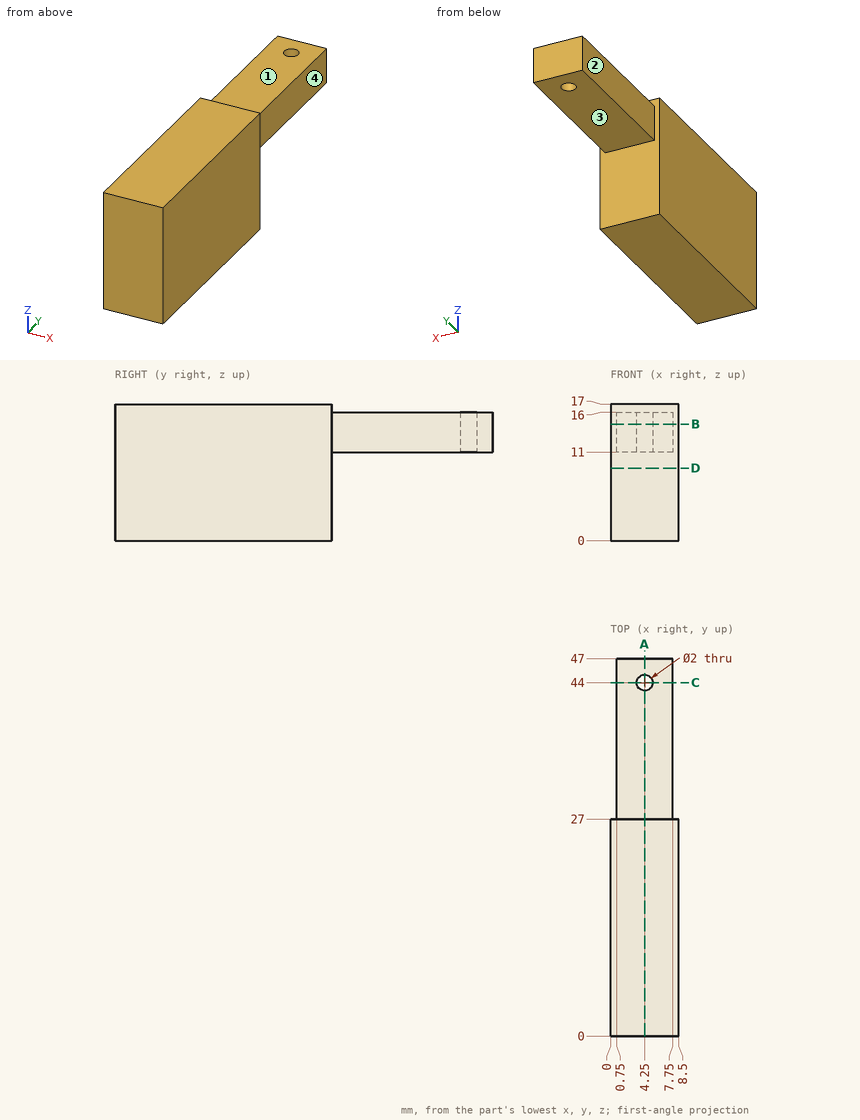
Answer from the drawing. Dimensions are ordinates in mm from the lowest x, y and z of the part. A direction names the side the tool comes from. Give positions to 0.01 mm unless a question says otherwise; leave off trailing zeros. Write each loop counter-clockwise with the first axis right and the second up, starting at its lowest first coordinate (ties: lowest second). Pieces come first, ordered by that corner, then holes. Notation, with made-up numbers: (75, -39.75) - (117, -39.75) arc R36 ccw to (117, -5.75) - close; hole circle Ø3 at (38, -23). An arc over 180 degrees is marked (long way). One line per item, written item: value. Start each with the question number.
1. Find section A-A (x = 4.25). Write down the section's boundary in (y, z), then the cut area to 3 significant figures.
2. Find section C-C (y = 44). Write down the section's boundary in (x, z), then the cut area to 3 significant figures.
3. Find section B-B (z = 14.5). Write down the section's boundary in (x, y).
4. Find section D-D (z = 9). Write down the section's boundary in (x, y).
5. Consider probe 1 along Y at (x, z) = (4.25, 13.3); probe 2 along Z at (x, y) = (7.25, 38.5); probe 3 along Y at (x, z) = (4.25, 1.5). Determine where each line is inside the solid, lowest interval first.
6. For the marked faces 1, 2, 3 and 4, determine the directions among +Z, -Z, +X, -X, +Y, -Y from which every point of the face is accessible in a straight line to the end or side of a thin tool.
7. Given pin 1 (1 mm diameter, centred on x = 5.5, y = 5, fed in from -Z); pin 2 (4 mm diameter, centred on x = 3.5, z = 8.5, fed in from +Y); pin 3 (4 mm diameter, centred on x = 4, y = 30, fed in from +Z); pin 4 (1.5 mm diameter, centred on y = 37.5, z = 13, fed in from -X), each flat-ended and moving along its own axis, determine where each tip first touches the part or whether it passes through.
Geometry results:
1. outline: (0, 0) - (27, 0) - (27, 11) - (43, 11) - (43, 16) - (27, 16) - (27, 17) - (0, 17) - close; (45, 11) - (47, 11) - (47, 16) - (45, 16) - close
1. area: 549 mm2
2. outline: (0.75, 11) - (3.25, 11) - (3.25, 16) - (0.75, 16) - close; (5.25, 11) - (7.75, 11) - (7.75, 16) - (5.25, 16) - close
2. area: 25.0 mm2
3. outline: (0, 0) - (8.5, 0) - (8.5, 27) - (7.75, 27) - (7.75, 47) - (0.75, 47) - (0.75, 27) - (0, 27) - close; hole circle Ø2 at (4.25, 44)
4. outline: (0, 0) - (8.5, 0) - (8.5, 27) - (0, 27) - close
5. probe 1: 0 to 43, 45 to 47
5. probe 2: 11 to 16
5. probe 3: 0 to 27
6. face 1: +Z, +X, -X, +Y
6. face 2: +Z, -Z, -X, +Y
6. face 3: -Z, +X, -X, +Y
6. face 4: +Z, -Z, +X, +Y
7. pin 1: z = 0
7. pin 2: y = 27
7. pin 3: z = 16
7. pin 4: x = 0.75
